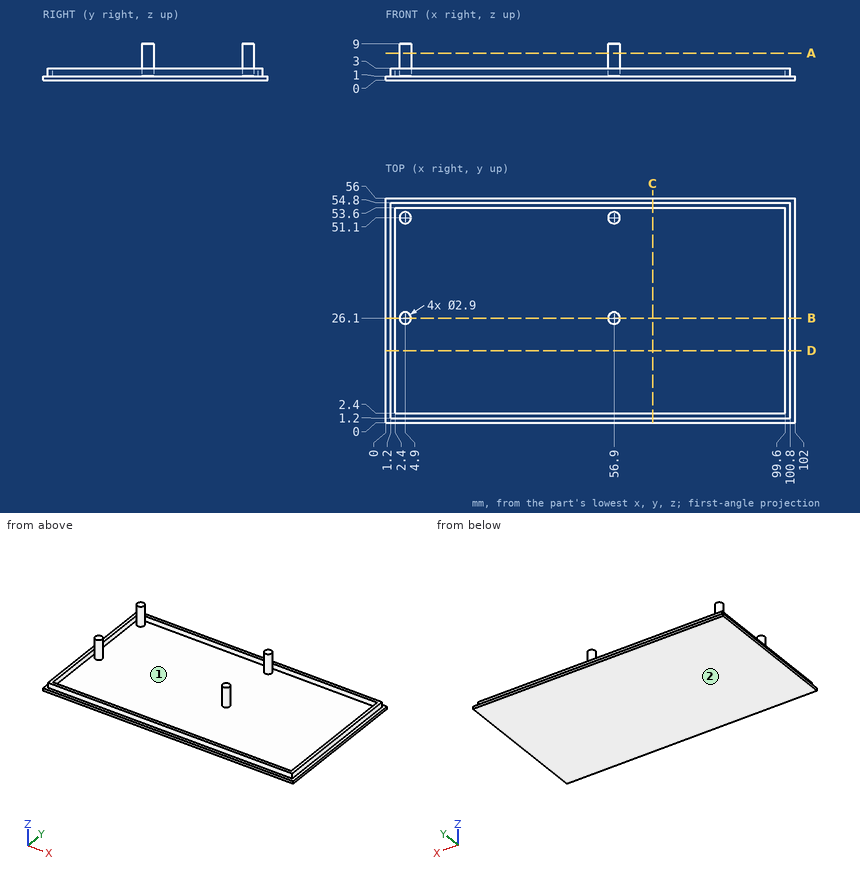
The drawing under review shows one solid part. Ordinate dimensions are in mm from its lowest x, y, z. Round coordinates to 2 decimals unless told otherwise and drop trailing zeros. Write each loop counter-clockwise with the first axis right and the second up, starting at its lowest first coordinate (ties: lowest second). Pieces come first, ordered by that corner, then holes. Notation, with made-up numbers: (8, 86) -> (38, 86) arc R33 cw to (38, 115) -> close; hole circle Ø10 at (74.25, -36). An arc over 180 degrees is marked (long way). Put each result on its own line as item: value.
Q1. Consider section B-B on y = 26.1. State the section outline as (x, z) points.
Determined:
outline: (0, 0) -> (102, 0) -> (102, 1) -> (100.8, 1) -> (100.8, 3) -> (99.6, 3) -> (99.6, 1) -> (58.35, 1) -> (58.35, 9) -> (55.45, 9) -> (55.45, 1) -> (6.35, 1) -> (6.35, 9) -> (3.45, 9) -> (3.45, 1) -> (2.4, 1) -> (2.4, 3) -> (1.2, 3) -> (1.2, 1) -> (0, 1) -> close
Q2. Clearance check with flat-ended pins moving along their axes: pin 1 Ø1 at (x, z) = (26, 2) entering from +Y; pin 2 Ø15.5 at (x, y) = (49.5, 38) entering from +Z; pin 3 Ø0.6 at (y, z) = (15, 1.5) entering from +X; pin 4 Ø3 at (y, z) = (41, 2) entering from +X. State where each tip first meets the part, or that it passes through.
Determined:
pin 1: stops at y = 54.8
pin 2: stops at z = 1
pin 3: stops at x = 100.8
pin 4: stops at x = 102
Q3. Consider section D-D on y = 18. State the section outline as (x, z) points.
Determined:
outline: (0, 0) -> (102, 0) -> (102, 1) -> (100.8, 1) -> (100.8, 3) -> (99.6, 3) -> (99.6, 1) -> (2.4, 1) -> (2.4, 3) -> (1.2, 3) -> (1.2, 1) -> (0, 1) -> close
Q4. Consider section A-A on z = 6.75. State the section outline as (x, y) points.
Determined:
outline: circle Ø2.9 at (4.9, 26.1); circle Ø2.9 at (4.9, 51.1); circle Ø2.9 at (56.9, 26.1); circle Ø2.9 at (56.9, 51.1)
Q5. The part is to be moulded in two halves that separate along X. For the marked faces 1 and 2, say which applies: released by +X, released by -X, zero draft, split by the parting line, or undercut.
Determined:
face 1: undercut
face 2: zero draft
Q6. To check wall thickness, follow L1, parallel to X at y = 36, z = 1.5; L2, parallel to Y at x = 85, z = 2.25; L3, parallel to Z at x = 13, y = 28. State the ranges of each line that lie inside material, in increasing order. Write a range as [from, to].
Determined:
L1: x = [1.2, 2.4], [99.6, 100.8]
L2: y = [1.2, 2.4], [53.6, 54.8]
L3: z = [0, 1]
Q7. Consider section C-C on x = 66.5. State the section outline as (y, z) points.
Determined:
outline: (0, 0) -> (56, 0) -> (56, 1) -> (54.8, 1) -> (54.8, 3) -> (53.6, 3) -> (53.6, 1) -> (2.4, 1) -> (2.4, 3) -> (1.2, 3) -> (1.2, 1) -> (0, 1) -> close
